Model file for the job. Use its own axes, mm. A direction names the side the tool comes from. Round coordinates to 2 decimals unless told otherwise and drop trailing zeros. Order: outer loops, then holes, each group sorted by start corner. A loop starts at its lowest first (then second) coordinate and runs counter-clockwise, first axis right, second up. Notation, with made-up numbers: (8.5, -32) - (58.5, -32) arc R23 ccw to (58.5, 1) - close; hole circle Ø8 at (85.25, 54.5). An arc over 180 degrees is marked (long way). Use one line per item in the form item = value.
from build123d import *

# Parameters (mm, degrees)
SKETCH1_W           = 33
SKETCH1_H           = 20
SKETCH1_R           = 1.4
BOSS_EXTRUDE1_DEPTH = 1.57
SKETCH2_W           = 5
SKETCH2_H           = 12
BOSS_EXTRUDE2_DEPTH = 1.5


with BuildPart() as part:
    # Sketch1 → Boss-Extrude1 (new body)
    with BuildSketch(Plane.YZ):
        Rectangle(SKETCH1_W, SKETCH1_H)
        with Locations(Location((12.75, 7.5, 0), (0, 0, 270))):
            Circle(SKETCH1_R, mode=Mode.SUBTRACT)
        with Locations(Location((12.75, -7.5, 0), (0, 0, 270))):
            Circle(SKETCH1_R, mode=Mode.SUBTRACT)
    extrude(amount=BOSS_EXTRUDE1_DEPTH)

    # Sketch2 → Boss-Extrude2 (add)
    with BuildSketch(Plane.YZ.offset(1.57)):
        Rectangle(SKETCH2_W, SKETCH2_H)
    extrude(amount=BOSS_EXTRUDE2_DEPTH)


solid = part.part
(1) Slice it at D-D on z = -3.75. Give the cut face in (x, y), then the cut area to 3 significant figures.
Report:
outline = (0, -16.5) - (1.57, -16.5) - (1.57, -2.5) - (3.07, -2.5) - (3.07, 2.5) - (1.57, 2.5) - (1.57, 16.5) - (0, 16.5) - close
area = 59.3 mm2
(2) Pull direction Z, two halves, no side cores. Call faces 4 (the face through (1, -16.5, 0)), 5 (the face through (0.77, 14.14, -7.32)), 6 (the face through (2, 0, 6)): released by +Z, released by -Z, zero draft, split by the parting line, or undercut.
Report:
face_4 = zero draft
face_5 = undercut
face_6 = released by +Z
(3) Slice it at B-B on z = -7.5. Give the cut face in (x, y), then the cut area to 3 significant figures.
Report:
outline = (0, -16.5) - (1.57, -16.5) - (1.57, 11.35) - (0, 11.35) - close; (0, 14.15) - (1.57, 14.15) - (1.57, 16.5) - (0, 16.5) - close
area = 47.4 mm2
(4) Probe probe 1 along Y at (x, z) = (0.7, 7.5); probe 2 along X at (y, z) = (4.5, -5); probe 3 along Y at (x, z) = (1.7, 4). List the from-to ranges inside material, lowest first. Write a range as [from, to].
Report:
probe_1 = [-16.5, 11.35], [14.15, 16.5]
probe_2 = [0, 1.57]
probe_3 = [-2.5, 2.5]
(5) Slice it at C-C on x = 1. Give the cut face in (y, z).
Report:
outline = (-16.5, -10) - (16.5, -10) - (16.5, 10) - (-16.5, 10) - close; hole circle Ø2.8 at (12.75, -7.5); hole circle Ø2.8 at (12.75, 7.5)
(6) Tool access for faces 1 (the face through (2, 0, -6)), 2 (the face through (2, -2.5, 0)), 3 (the face through (2, 2.5, 0)): list every direction of +Z, -Z, +X, -X, +Y, -Y with a clear straight run to the whole face (end or side of a thin tool).
Report:
face_1 = -Z, +X, +Y, -Y
face_2 = +Z, -Z, +X, -Y
face_3 = +Z, -Z, +X, +Y
(7) Slice it at A-A on y = 12.75. Give the cut face in (x, z).
Report:
outline = (0, -10) - (1.57, -10) - (1.57, -8.9) - (0, -8.9) - close; (0, -6.1) - (1.57, -6.1) - (1.57, 6.1) - (0, 6.1) - close; (0, 8.9) - (1.57, 8.9) - (1.57, 10) - (0, 10) - close
(8) Pin check, flat tips, straight feed: pin 1 (3 mm diameter, centred on y = 12.75, z = 7.5, fed in from +X); pin 2 (0.5 mm diameter, centred on x = 2, y = 0.5, fed in from +Z); pin 3 (0.8 mm diameter, centred on x = 2, z = -1, fed in from -Y). Stop position of each tip, or through.
Report:
pin_1 = 1.57
pin_2 = 6
pin_3 = -2.5
